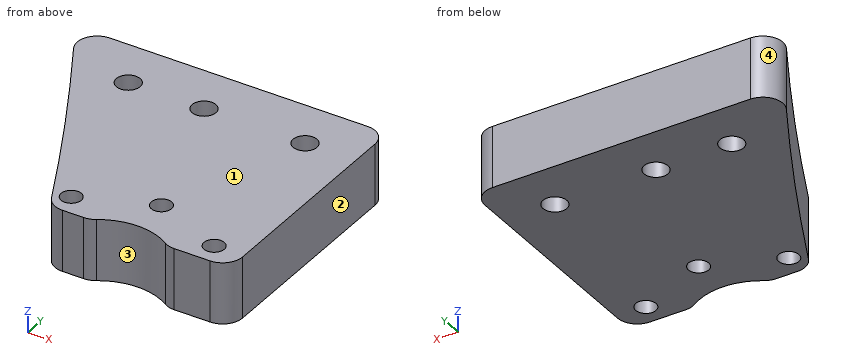
Autodesk Inventor part; units mm, degrees
ref_plane "YZ Plane" through (0, 0, 0) normal (1, 0, 0) x (0, 1, 0)
ref_plane "XZ Plane" through (0, 0, 0) normal (0, 1, 0) x (-1, 0, 0)
ref_plane "XY Plane" through (0, 0, 0) normal (0, 0, 1) x (1, 0, 0)
sketch "Sketch1" plane through (0, 0, 0) normal (0, 0, 1) x (1, 0, 0)
  line L0 (-110, -20.8494) -> (-110, 0)
  line L1 (-110, 0) -> (0, 0)
  line L2 (0, 0) -> (0, -105)
  line L3 (0, -105) -> (-39.3892, -105)
  line L4 (-110, -20.8494) -> (-119.38, 0) construction
  line L5 (-119.38, 0) -> (-110, 0) construction
  line L6 (-50.8, -25.4) -> (0, -25.4) construction
  line L7 (0, -25.4) -> (0, 0) construction
  line L8 (0, 0) -> (-50.8, 0) construction
  line L9 (-50.8, 0) -> (-50.8, -25.4) construction
  line L10 (-50.8, -25.4) -> (0, 0) construction
  line L11 (0, -25.4) -> (-50.8, 0) construction
  circle A0 centre (-12.7, -12.7) radius 3
  circle A1 centre (-38.1, -12.7) radius 3
  circle A2 centre (-25.4, -75) radius 15.875
  circle A3 centre (-25.4, -75) radius 30
  line L12 (-50.8, -90.9637) -> (-50.8, -59.0363)
  line L13 (-110, -4.7091) -> (-83.2932, 0)
  arc A4 (-56.3982, -84.7295) -> (-61.7755, -78.3211) centre (-62.3821, -84.2903) ccw
  line L14 (-39.3892, -105) -> (-56.3982, -84.7295)
  arc A5 (-85.9963, -49.4559) -> (-100.0831, -32.6679) centre (-102.5, -49) ccw
  line L15 (-61.7755, -78.3211) -> (-85.9963, -49.4559)
  line L16 (-100.0831, -32.6679) -> (-110, -20.8494)
  circle A6 centre (-95.25, -12.7) radius 3
  circle A7 centre (-57.15, -12.7) radius 3
  point P0 (0, 0)
  point P1 (-25.4, -12.7)
  point P2 (-25.4, -25.4)
  point P3 (-50.8, -75)
  point P4 (0, -90.9637)
  point P5 (-110, -10.4247)
  point P6 (-48.3813, -94.2836)
  point P7 (0, -59.0363)
  point P8 (-25.4, -105)
  dimension "d1" = 119.38
  dimension "d2" = 50.8
  dimension "d3" = 25.4
  dimension "d4" = 25.4
  dimension "d5" = 12.7
  dimension "d6" = 6
  dimension "d7" = 6
  dimension "d11" = 110
  dimension "d12" = 60
  dimension "d13" = 25.4
  dimension "d14" = 25.4
  dimension "d17" = 20.8494
  dimension "d18" = 31.75
  dimension "d21" = 170
  dimension "d22" = 26.7068
  dimension "d24" = 86.6409
  dimension "d25" = 12
  dimension "d26" = 47.6179
  dimension "d28" = 81.3659
  dimension "d29" = 33.02
  dimension "d30" = 49
  dimension "d31" = 50
  dimension "d41" = 19.05
  dimension "d42" = 38.1
extrude "Extrusion1" add sketch "Sketch1" along normal blind 15.4305 contours L0 L13 L1 L2 A3 L14 A4 L15 A5 L16 | L2 A3 L12 | L12 A3
fillet "Fillet1" radius 6 8 edges at (0, -90.9637, 7.7153) (-110, -20.8494, 7.7153) (-110, -4.7091, 7.7153) (-83.2932, 0, 7.7153) (-56.3982, -84.7295, 7.7153) (-61.7755, -78.3211, 7.7153) (-85.9963, -49.4559, 7.7153) (-100.0831, -32.6679, 7.7153)
sketch "Sketch2" plane through (0, 0, 0) normal (0, 0, -1) x (-1, 0, 0)
  circle A0 centre (25.4, -75) radius 15.875
  circle A1 centre (25.4, -75) radius 25.4
  line L0 (7.4395, -92.9605) -> (7.4395, -57.0395)
  line L1 (43.3605, -57.0395) -> (43.3605, -92.9605)
  line L2 (7.4395, -92.9605) -> (25.4, -75)
  line L3 (25.4, -75) -> (43.3605, -57.0395)
  point P0 (0, 0)
  point P1 (25.4, -100.4)
  point P2 (25.4, -49.6)
  dimension "d32" = 50.8
  dimension "d33" = 45
hole "Hole1" at (-7.4395, -92.9605, 0) at (-7.4395, -57.0395, 0) at (-43.3605, -57.0395, 0) at (-43.3605, -92.9605, 0) at (-25.4, -100.4, 0) at (-25.4, -49.6, 0) direction (0, 0, 1) diameter 5.105 end through all
sketch "Sketch3" plane through (0, 0, 0) normal (0, 0, -1) x (-1, 0, 0)
  circle A0 centre (25.4, -49.6) radius 2.5525 construction
  circle A1 centre (25.4, -100.4) radius 2.5525 construction
  circle A2 centre (43.3605, -92.9605) radius 2.5525 construction
  circle A3 centre (43.3605, -57.0395) radius 2.5525 construction
  circle A4 centre (7.4395, -57.0395) radius 2.5525 construction
  circle A5 centre (7.4395, -92.9605) radius 2.5525 construction
  arc A6 (98.3371, -33.0234) -> (101.4205, -31.074) centre (96.8242, -27.2173) ccw construction
  line L0 (108.5963, -22.5223) -> (101.4205, -31.074) construction
  arc A7 (108.5963, -22.5223) -> (110, -18.6655) centre (104, -18.6655) ccw construction
  line L1 (110, -9.7437) -> (110, -18.6655) construction
  arc A8 (110, -9.7437) -> (105.0419, -3.8349) centre (104, -9.7437) ccw construction
  line L2 (83.8101, -0.0912) -> (105.0419, -3.8349) construction
  arc A9 (83.8101, -0.0912) -> (82.7682, 0) centre (82.7682, -6) ccw construction
  line L3 (0, 0) -> (82.7682, 0)
  line L4 (0, -89.1294) -> (0, 0)
  arc A10 (0, -89.1294) -> (1.15, -92.6618) centre (6, -89.1294) ccw construction
  arc A11 (1.15, -92.6618) -> (48.3813, -94.2836) centre (25.4, -75) ccw construction
  line L5 (55.1309, -86.2398) -> (48.3813, -94.2836) construction
  arc A12 (55.1309, -86.2398) -> (56.4584, -83.3367) centre (50.5346, -82.3831) ccw construction
  arc A13 (60.4143, -78.6222) -> (56.4584, -83.3367) centre (62.3821, -84.2903) ccw construction
  arc A14 (60.4143, -78.6222) -> (63.0428, -76.8108) centre (58.4465, -72.954) ccw construction
  line L6 (84.6589, -51.0497) -> (63.0428, -76.8108) construction
  arc A15 (84.6589, -51.0497) -> (86.0433, -47.6746) centre (80.0627, -47.193) ccw construction
  arc A16 (98.3371, -33.0234) -> (86.0433, -47.6746) centre (102.5, -49) ccw construction
  circle A17 centre (25.4, -75) radius 15.875 construction
  circle A18 centre (38.1, -12.7) radius 3 construction
  circle A19 centre (12.7, -12.7) radius 3 construction
  circle A20 centre (95.25, -12.7) radius 3 construction
  circle A21 centre (57.15, -12.7) radius 3 construction
  line L7 (0, -62.5) -> (45.2947, -62.5)
  arc A22 (78.5605, 0) -> (45.2947, -62.5) centre (770.086, -408.1685) ccw
  arc A23 (75.8423, -7.7632) -> (9.6381, -155.1512) centre (770.086, -408.1685) ccw construction
  point P0 (0, 0)
  dimension "d43" = 803
  dimension "d44" = 62.5
extrude "Extrusion2" cut sketch "Sketch3" along normal through all both and the other way through all keep common part
fillet "Fillet2" radius 5 6 edges at (-78.5605, 0, 7.7153) (-45.2947, -62.5, 7.7153) (-15.614, -62.5, 7.7153) (-35.186, -62.5, 7.7153) (0, -62.5, 7.7153) (0, 0, 7.7153)
equation "\"d7\" = d6"
properties part number "SPACER,INTAKE,LINEAR" material "3D Print Material - chopped carbon Nylon12 (preferred)"
Work out the finished part from the listing and answer in its coordinate system (mm). Face numbers are marked on the shaded views. Coordinates: 2 decimals unless noted, no trailing zeros. Order: outer loops, then holes, each group sorted by start corner. A loop starts at its lowest first (then second) coordinate and runs counter-clockwise, first axis right, second up. Notation, with made-up numbers: (16, 3.25) - (72, 3.25) arc R28 ccw to (72, 36.25) - close; hole circle Ø3 at (-11, 84). An arc over 180 degrees is marked (long way). Put each result on its own line as item: value. Start each with the question number.
1) Find section D-D (z = 7.75). State how many separate pieces and enclosed holes the cut face has, plus the area to 3 significant figures.
2) Find section A-A (y = -12.7). Give the vertices of the cut face in (x, z), plus the area to 3 significant figures.
3) Find section C-C (y = -56). Give the vertices of the cut face in (x, z).
4) Find section B-B (x = -12.7). Give the vertices of the cut face in (y, z), plus the area to 3 significant figures.
5) Find the intervals of material crossed by line 1 (Y direction, x = -38.1, z = 5.25); line 2 (X direction, y = -55, z = 9.5); line 3 (Y direction, x = -57.15, z = 10.25), in increasing order. Write a range as from..to.
6) Flat-ended cylindrical pins translate along their axes: pin 1 (8 mm diameter, centred on x = -38.1, y = -12.7, fed in from -Z); pin 2 (1 mm diameter, centred on y = -22.5, z = 13, fed in from -X); pin 3 (1 mm diameter, centred on y = -30.5, z = 12, fed in from -X). Find the tip coordinate at first contact, or state that the pin passes through.
7) For a pull along X with two mould halves and no side action, classify the marked faces 1, 2, 3 and 4 as released by +X, released by -X, zero draft, split by the parting line, or undercut.
Results list:
1. separate pieces: 1
1. enclosed holes: 6
1. area: 3,610 mm^2
2. outline: (-71.22, 0) - (-60.15, 0) - (-60.15, 15.43) - (-71.22, 15.43) - close; (-54.15, 0) - (-41.1, 0) - (-41.1, 15.43) - (-54.15, 15.43) - close; (-35.1, 0) - (-15.7, 0) - (-15.7, 15.43) - (-35.1, 15.43) - close; (-9.7, 0) - (0, 0) - (0, 15.43) - (-9.7, 15.43) - close
2. area: 821 mm^2
3. outline: (-48.43, 0) - (-45.69, 0) - (-45.69, 15.43) - (-48.43, 15.43) - close; (-41.03, 0) - (-9.77, 0) - (-9.77, 15.43) - (-41.03, 15.43) - close; (-5.11, 0) - (0, 0) - (0, 15.43) - (-5.11, 15.43) - close
4. outline: (-62.5, 0) - (-15.7, 0) - (-15.7, 15.43) - (-62.5, 15.43) - close; (-9.7, 0) - (0, 0) - (0, 15.43) - (-9.7, 15.43) - close
4. area: 872 mm^2
5. line 1: y = -62.5..-15.7, -9.7..0
5. line 2: x = -48.92..-44.9, -41.83..-8.97, -5.9..0
5. line 3: y = -38.67..-15.7, -9.7..0
6. pin 1: stops at z = 0
6. pin 2: stops at x = -66.04
6. pin 3: stops at x = -61.71
7. face 1: zero draft
7. face 2: released by +X
7. face 3: undercut
7. face 4: released by -X
